The model under review builds one solid part; all positions refer to its coordinate system, in mm. A direction names the side the tool comes from. Give positions to 0.01 mm unless a question says otherwise; leave off trailing zeros. Loops run counter-clockwise (first coordinate to the right, second up) from the corner with the lowest first, then second, coordinate; pieces in that order, holes last. Notation, with made-up numbers: (-22.5, 3) -> (8.5, 3) arc R26 cw to (8.5, 36) -> close; hole circle Ø6 at (39, 51.5). An arc over 180 degrees is marked (long way). Write each question's results on one line, items separated by ' | '. Start each with the question number.
Q1. Mouldability with a two-part tool opening along X and no side actions: class faces 4 (the face through (129.86, 17.94, 2.12)), 5 (the face through (46.596, -19, 2)), 6 (the face through (-110.32, -6.17, 2.12)) as released by +X, released by -X, zero draft, split by the parting line, or undercut.
Q2. Machinability: for faces 1 (the face through (-1, 19.05, 2)), 2 (the face through (-129.86, 17.94, 2.12)), 3 (the face through (-64, -11.43, 2)), which of the approach directions +Z, -Z, +X, -X, +Y, -Y give a long, thin tool a straight path to every point of the face, cutting with its end or side? Answer none if there is none.
Q3. We need section A-A (x = 118). Write out the cut boundary in (y, z), plus the area to 3 significant figures.
Q4. Wall thickness on L1, parallel to Y at x = 64, z = 0.8; L2, parallel to Y at x = 38.5, z = 2.35; L3, parallel to X at y = 23, z = 1.2: over which ranges is each line inside the solid? List them lowest first. Write a range as [from, to].
Q5. Insertion check: pin 1 Ø2 at (x, z) = (-64, 2) entering from -Y; pin 2 Ø2 at (y, z) = (-20, 1) entering from -X; pin 3 Ø1.3 at (y, z) = (-19, 1.5) entering from +X. Each pin has a flat end and moves straight along its axis. Give the tip position at first contact, or say it passes through.
Q6. We need section B-B (y = 14). Write out the cut boundary in (x, z), plus the area to 3 significant figures.
from build123d import *

# Parameters (mm, degrees)
SKETCH1_W           = 152.4
SKETCH1_H           = 38.1
BOSS_EXTRUDE1_DEPTH = 4.2926
SKETCH3_W           = 4.2926
SKETCH3_H           = 20.32
CUT_EXTRUDE2_DEPTH  = 4.2926


with BuildPart() as part:
    # Sketch1 → Boss-Extrude1 (new body)
    with BuildSketch(Plane.XY):
        Polygon((-83.82, 29.21), (-134.62, 29.21), (-124.968, 6.35), (-95.25, -19.05), (-76.2, -19.05), (-76.2, 19.05), align=None)
        Rectangle(SKETCH1_W, SKETCH1_H)
        with BuildLine():
            Line((-76.2, -19.05), (-95.25, -19.05))
            add(Edge.make_bspline(
                [(-95.25, -19.05), (-66.079235011, -25.514680938), (-2.12159074, -32.083739423), (61.761861898, -25.010246771), (95.25, -19.05)],
                knots=[0, 0, 0, 0, 0.467198678, 1, 1, 1, 1], degree=3))
            Line((95.25, -19.05), (76.2, -19.05))
            Line((76.2, -19.05), (-76.2, -19.05))
        make_face()
        Polygon((95.25, -19.05), (76.2, -19.05), (76.2, 19.05), (83.82, 29.21), (134.62, 29.21), (124.968, 6.35), align=None)
    extrude(amount=BOSS_EXTRUDE1_DEPTH)

    # Sketch3 → Cut-Extrude2 (cut)
    with BuildSketch(Plane.XY.offset(4.2926)):
        with Locations((-63.5, -21.59)):
            Rectangle(SKETCH3_W, SKETCH3_H)
        with Locations((-44.45, -21.59)):
            Rectangle(SKETCH3_W, SKETCH3_H)
        with Locations((-19.05, -21.59)):
            Rectangle(SKETCH3_W, SKETCH3_H)
        with Locations((44.45, -21.59)):
            Rectangle(SKETCH3_W, SKETCH3_H)
        with Locations((63.5, -21.59)):
            Rectangle(SKETCH3_W, SKETCH3_H)
        with Locations((19.05, -21.59)):
            Rectangle(SKETCH3_W, SKETCH3_H)
    extrude(amount=-CUT_EXTRUDE2_DEPTH, mode=Mode.SUBTRACT)


solid = part.part
Output:
1) face 4: released by +X | face 5: undercut | face 6: released by -X
2) face 1: +Z, -Z, +Y | face 2: +Z, -Z, -X, -Y | face 3: +Z, -Z, -Y
3) outline: (0.39, 0) -> (29.21, 0) -> (29.21, 4.29) -> (0.39, 4.29) -> close | area: 124 mm2
4) L1: [-11.43, 19.05] | L2: [-26.71, 19.05] | L3: [-132, -79.16], [79.16, 132]
5) pin 1: y = -11.43 | pin 2: x = -95.31 | pin 3: x = 96.07
6) outline: (-128.2, 0) -> (128.2, 0) -> (128.2, 4.29) -> (-128.2, 4.29) -> close | area: 1,100 mm2
